The listing builds one solid part. Answer for the finished solid, in the listing's coordinates (mm). Face numbers are marked on the shaded views. A direction names the side the tool comes from. Give positions to 0.01 mm unless a question says otherwise; leave off trailing zeros. Loops run counter-clockwise (first coordinate to the right, second up) from the corner with the lowest first, then second, coordinate; pieces in that order, holes last. Notation, with made-up numbers: (82.25, 43) - (111.25, 43) arc R34 cw to (111.25, 80) - close; hole circle Ø2 at (72, 56). An arc over 180 degrees is marked (long way). One line per item, written item: value. Start each with the question number.
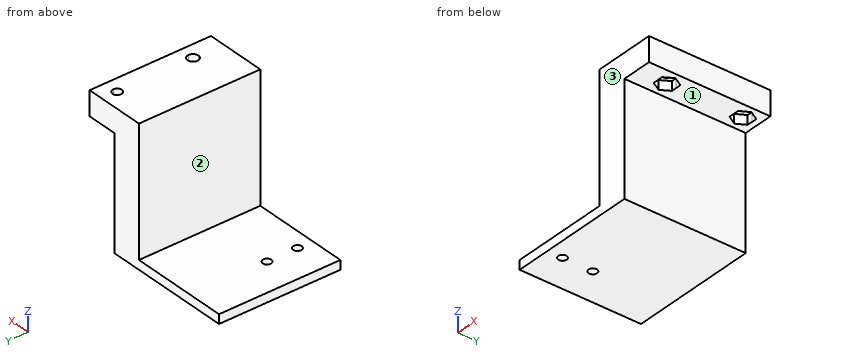
from build123d import *

# Parameters (mm, degrees)
SKETCH1_W           = 10
SKETCH1_H           = 40
BOSS_EXTRUDE1_DEPTH = 5
SKETCH1_4_W         = 10
SKETCH1_4_H         = 40
BOSS_EXTRUDE2_DEPTH = 3
BOSS_EXTRUDE3_START = 5
SKETCH1_5_W         = 10
SKETCH1_5_H         = 40
BOSS_EXTRUDE3_DEPTH = 44.8
BOSS_EXTRUDE4_START = -39.8
SKETCH1_6_W         = 22.5
SKETCH1_6_H         = 40
SKETCH1_6_R         = 1.4
SKETCH1_6_W_2       = 10
BOSS_EXTRUDE4_DEPTH = 3


with BuildPart() as part:
    # Sketch1 → Boss-Extrude1 (new body)
    with BuildSketch(Plane.XY):
        Polygon((54.918901731, 32.442311257), (49.918901731, 32.442311257), (49.918901731, 30.44249106), (51.6180048, 30.461093919), (53.382795739, 27.480236167), (51.683692671, 24.461453505), (49.918901731, 24.442131453), (49.918901731, 5.44249106), (51.683692671, 5.423169009), (53.382795739, 2.404386347), (51.6180048, -0.576471406), (49.918901731, -0.557868547), (49.918901731, -7.557688743), (54.918901731, -7.557688743), align=None)
        Polygon((49.918901731, 32.442311257), (44.918901731, 32.442311257), (44.918901731, -7.557688743), (49.918901731, -7.557688743), (49.918901731, -0.557868547), (48.154110791, -0.538546495), (46.455007723, 2.480236167), (48.219798662, 5.461093919), (49.918901731, 5.44249106), (49.918901731, 24.442131453), (48.219798662, 24.423528594), (46.455007723, 27.404386347), (48.154110791, 30.423169009), (49.918901731, 30.44249106), align=None)
        with BuildLine():
            Line((49.918901731, 0.655890403), (49.918901731, -0.557868547))
            Line((49.918901731, -0.557868547), (51.6180048, -0.576471406))
            Line((51.6180048, -0.576471406), (53.382795739, 2.404386347))
            Line((53.382795739, 2.404386347), (51.683692671, 5.423169009))
            Line((51.683692671, 5.423169009), (49.918901731, 5.44249106))
            Line((49.918901731, 5.44249106), (49.918901731, 4.22873211))
            ThreePointArc((49.918901731, 4.22873211), (51.182092031, 3.705501556), (51.705322585, 2.442311257))
            ThreePointArc((51.705322585, 2.442311257), (51.182092031, 1.179120957), (49.918901731, 0.655890403))
        make_face()
        with BuildLine():
            Line((48.154110791, -0.538546495), (49.918901731, -0.557868547))
            Line((49.918901731, -0.557868547), (49.918901731, 0.655890403))
            ThreePointArc((49.918901731, 0.655890403), (48.132480877, 2.442311257), (49.918901731, 4.22873211))
            Line((49.918901731, 4.22873211), (49.918901731, 5.44249106))
            Line((49.918901731, 5.44249106), (48.219798662, 5.461093919))
            Line((48.219798662, 5.461093919), (46.455007723, 2.480236167))
            Line((46.455007723, 2.480236167), (48.154110791, -0.538546495))
        make_face()
        with BuildLine():
            Line((51.6180048, 30.461093919), (49.918901731, 30.44249106))
            Line((49.918901731, 30.44249106), (49.918901731, 28.967240827))
            ThreePointArc((49.918901731, 28.967240827), (50.997189771, 28.520599297), (51.443831301, 27.442311257))
            ThreePointArc((51.443831301, 27.442311257), (50.997189771, 26.364023217), (49.918901731, 25.917381686))
            Line((49.918901731, 25.917381686), (49.918901731, 24.442131453))
            Line((49.918901731, 24.442131453), (51.683692671, 24.461453505))
            Line((51.683692671, 24.461453505), (53.382795739, 27.480236167))
            Line((53.382795739, 27.480236167), (51.6180048, 30.461093919))
        make_face()
        with BuildLine():
            Line((49.918901731, 28.967240827), (49.918901731, 30.44249106))
            Line((49.918901731, 30.44249106), (48.154110791, 30.423169009))
            Line((48.154110791, 30.423169009), (46.455007723, 27.404386347))
            Line((46.455007723, 27.404386347), (48.219798662, 24.423528594))
            Line((48.219798662, 24.423528594), (49.918901731, 24.442131453))
            Line((49.918901731, 24.442131453), (49.918901731, 25.917381686))
            ThreePointArc((49.918901731, 25.917381686), (48.39397216, 27.442311257), (49.918901731, 28.967240827))
        make_face()
        with Locations((39.918901731, 12.442311257)):
            Rectangle(SKETCH1_W, SKETCH1_H)
    extrude(amount=BOSS_EXTRUDE1_DEPTH)

    # Sketch1<4> → Boss-Extrude2 (add)
    with BuildSketch(Plane.XY):
        Polygon((49.918901731, 32.442311257), (44.918901731, 32.442311257), (44.918901731, -7.557688743), (49.918901731, -7.557688743), (49.918901731, -0.557868547), (48.154110791, -0.538546495), (46.455007723, 2.480236167), (48.219798662, 5.461093919), (49.918901731, 5.44249106), (49.918901731, 24.442131453), (48.219798662, 24.423528594), (46.455007723, 27.404386347), (48.154110791, 30.423169009), (49.918901731, 30.44249106), align=None)
        Polygon((54.918901731, 32.442311257), (49.918901731, 32.442311257), (49.918901731, 30.44249106), (51.6180048, 30.461093919), (53.382795739, 27.480236167), (51.683692671, 24.461453505), (49.918901731, 24.442131453), (49.918901731, 5.44249106), (51.683692671, 5.423169009), (53.382795739, 2.404386347), (51.6180048, -0.576471406), (49.918901731, -0.557868547), (49.918901731, -7.557688743), (54.918901731, -7.557688743), align=None)
        with Locations((39.918901731, 12.442311257)):
            Rectangle(SKETCH1_4_W, SKETCH1_4_H)
    extrude(amount=-BOSS_EXTRUDE2_DEPTH)

    # Sketch1<5> → Boss-Extrude3 (add)
    with BuildSketch(Plane.XY.offset(BOSS_EXTRUDE3_START)):
        with Locations((39.918901731, 12.442311257)):
            Rectangle(SKETCH1_5_W, SKETCH1_5_H)
    extrude(amount=-BOSS_EXTRUDE3_DEPTH)

    # Sketch1<6> → Boss-Extrude4 (add)
    with BuildSketch(Plane.XY.offset(BOSS_EXTRUDE4_START)):
        with Locations((13.668901731, 12.442311257)):
            Rectangle(SKETCH1_6_W, SKETCH1_6_H)
        with Locations((13.668901731, -2.557688743)):
            Circle(SKETCH1_6_R, mode=Mode.SUBTRACT)
        with Locations((13.668901731, 7.442311257)):
            Circle(SKETCH1_6_R, mode=Mode.SUBTRACT)
        with Locations((29.918901731, 12.442311257)):
            Rectangle(SKETCH1_6_W_2, SKETCH1_6_H)
    extrude(amount=BOSS_EXTRUDE4_DEPTH)


solid = part.part
1. A cutting plane is placed at A-A (z = 2.5). Determine the outline of the cut face in (x, y).
2. Flat-ended cylindrical pins translate along their axes: pin 1 (2 mm diameter, centred on x = 13.5, y = 19.5, fed in from +Z); pin 2 (1.8 mm diameter, centred on x = 50.5, y = 28.5, fed in from -Z); pin 3 (3 mm diameter, centred on x = 49, y = 4, fed in from -Z). Find the tip coordinate at first contact, or state that the pin passes through.
3. A cutting plane is placed at D-D (x = 27). Determine the outline of the cut face in (y, z).
4. Find the intervals of material crossed by L1, parallel to Z at x = 45.5, y = 2; L2, parallel to X at y = 22, z = 0.5; L3, parallel to Z at x = 8, y = 15, in increasing order. Write a range as [from, to].
5. A cutting plane is placed at B-B (y = 22.5). Determine the outline of the cut face in (x, z), plus the area to 4 significant figures.
6. For the marked faces 1, 2 and 3, determine the directions among +Z, -Z, +X, -X, +Y, -Y from which every point of the face is accessible in a straight line to the end or side of a thin tool.
7. A cutting plane is placed at C-C (x = 13.5). Determine the outline of the cut face in (y, z).
Results below:
1. outline: (34.92, -7.56) - (54.92, -7.56) - (54.92, 32.44) - (34.92, 32.44) - close; hole circle Ø3.57 at (49.92, 2.44); hole circle Ø3.05 at (49.92, 27.44)
2. pin 1: stops at z = -36.8
2. pin 2: stops at z = 0
2. pin 3: stops at z = -3
3. outline: (-7.56, -39.8) - (32.44, -39.8) - (32.44, -36.8) - (-7.56, -36.8) - close
4. L1: z = [-3, 5]
4. L2: x = [34.92, 54.92]
4. L3: z = [-39.8, -36.8]
5. outline: (2.42, -39.8) - (44.92, -39.8) - (44.92, -3) - (54.92, -3) - (54.92, 5) - (34.92, 5) - (34.92, -36.8) - (2.42, -36.8) - close
5. area: 625.5 mm^2
6. face 1: -Z, +X, +Y, -Y
6. face 2: +Z, -X, +Y, -Y
6. face 3: +Z, -Z, +X, -X, -Y
7. outline: (-7.56, -39.8) - (-3.95, -39.8) - (-3.95, -36.8) - (-7.56, -36.8) - close; (-1.17, -39.8) - (6.05, -39.8) - (6.05, -36.8) - (-1.17, -36.8) - close; (8.83, -39.8) - (32.44, -39.8) - (32.44, -36.8) - (8.83, -36.8) - close
